Design review of the part built by this model. Coordinates are the model's own, in mm. Face numbers are marked on the shaded views. A direction names the side the tool comes from. Coordinates: 2 decimals unless noted, no trailing zeros. Loops run counter-clockwise (first coordinate to the right, second up) from the corner with the lowest first, then second, coordinate; pieces in that order, holes last. Notation, with made-up numbers: (-13, -3.75) -> (6, -3.75) arc R37 cw to (6, 32.25) -> close; hole circle Ø2 at (-17.75, 15.5). An arc over 180 degrees is marked (long way). Use one line per item in the form item = value. Start each with the question number.
1. Wall thickness on line 1 (Y direction, x = -35, z = 1.4); line 2 (X direction, y = -2.5, z = 2.5); line 3 (X direction, y = 1, z = 4.5): over which ranges is each line inside the solid? List them lowest first. Write a range as from..to.
2. Consider section A-A (z = 3.5). State the section outline as (x, y) points (3 decimals).
3. For pin 1 (5 mm diameter, centred on x = 35, y = 0, fed in from +Z); pin 2 (1.5 mm diameter, centred on y = -1.5, z = 2.5, fed in from +X); pin 3 (1.5 mm diameter, centred on x = -34, z = 3.5, fed in from +Y); pin 4 (1 mm diameter, centred on x = 17.5, z = 4.5, fed in from +Y), all flat-tipped, find the tip position at first contact; note any pin that passes through.
4. Machinability: for the marked faces 4, 5 and 6, which of the approach directions +Z, -Z, +X, -X, +Y, -Y give a long, thin tool a straight path to every point of the face, cutting with its end or side? Answer none if there is none.
5. The part is to be moulded in two halves that separate along Y. For the marked faces 1, 2 and 3, say which applies: released by +Y, released by -Y, zero draft, split by the parting line, or undercut.
6. Consider section C-C (x = -6). State the section outline as (y, z) points.
7. Consider section B-B (y = 0). State the section outline as (x, z) points (3 decimals), then the cut area to 3 significant figures.
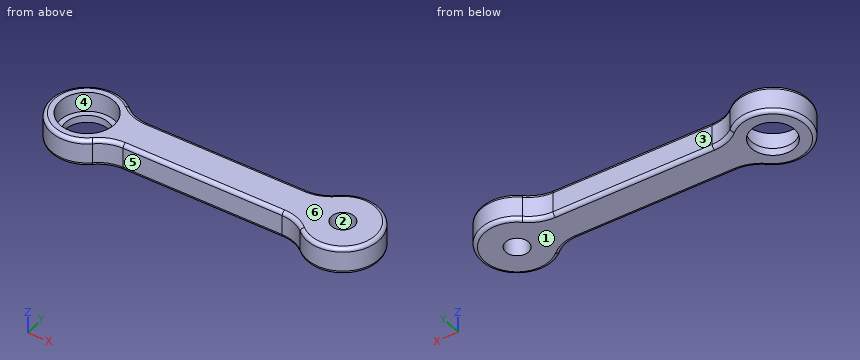
from build123d import *

# Parameters (mm, degrees)
BOSS_EXTRUDE1_DEPTH = 7.5
SKETCH2_R           = 7.5
CUT_EXTRUDE1_DEPTH  = 5.5
SKETCH3_R           = 6
CUT_EXTRUDE2_DEPTH  = 3
SKETCH4_R           = 3.175
CUT_EXTRUDE3_DEPTH  = 8.5
FILLET1_R           = 1


with BuildPart() as part:
    # Sketch1 → Boss-Extrude1 (new body)
    with BuildSketch(Plane.XY):
        with BuildLine():
            Line((-21.771243445, 5), (21.771243445, 5))
            ThreePointArc((21.771243445, 5), (25.306777351, 5.645856533), (28.385621722, 7.5))
            ThreePointArc((28.385621722, 7.5), (45, 0), (28.385621722, -7.5))
            ThreePointArc((28.385621722, -7.5), (25.306777351, -5.645856533), (21.771243445, -5))
            Line((21.771243445, -5), (-21.771243445, -5))
            ThreePointArc((-21.771243445, -5), (-25.306777351, -5.645856533), (-28.385621722, -7.5))
            ThreePointArc((-28.385621722, -7.5), (-45, 0), (-28.385621722, 7.5))
            ThreePointArc((-28.385621722, 7.5), (-25.306777351, 5.645856533), (-21.771243445, 5))
        make_face()
    extrude(amount=BOSS_EXTRUDE1_DEPTH)

    # Sketch2 → Cut-Extrude1 (cut)
    with BuildSketch(Plane.XY.offset(7.5)):
        with Locations((-35, 0)):
            Circle(SKETCH2_R)
    extrude(amount=-CUT_EXTRUDE1_DEPTH, mode=Mode.SUBTRACT)

    # Sketch3 → Cut-Extrude2 (cut, through all)
    with BuildSketch(Plane.XY.offset(2)):
        with Locations((-35, 0)):
            Circle(SKETCH3_R)
    extrude(amount=-CUT_EXTRUDE2_DEPTH, mode=Mode.SUBTRACT)

    # Sketch4 → Cut-Extrude3 (cut, through all)
    with BuildSketch(Plane(origin=(0, 0, 0), x_dir=(-1, 0, 0), z_dir=(0, 0, -1))):
        with Locations((-35, 0)):
            Circle(SKETCH4_R)
    extrude(amount=-CUT_EXTRUDE3_DEPTH, mode=Mode.SUBTRACT)

    # Fillet1
    fillet1_edges = [part.edges().sort_by_distance(p)[0] for p in [
        (25.306777351, 5.645856533, 7.5),
        (45, 0, 0),
        (25.306777351, -5.645856533, 0),
        (0, 5, 7.5),
        (-25.306777351, 5.645856533, 7.5),
        (-45, 0, 7.5),
        (-25.306777351, -5.645856533, 7.5),
        (0, -5, 7.5),
        (25.306777351, -5.645856533, 7.5),
        (45, 0, 7.5),
        (0, -5, 0),
        (-25.306777351, -5.645856533, 0),
        (-45, 0, 0),
        (-25.306777351, 5.645856533, 0),
        (0, 5, 0),
        (25.306777351, 5.645856533, 0),
    ]]
    fillet(fillet1_edges, radius=FILLET1_R)


solid = part.part
Geometry check:
q1.line_1 = -10..-6, 6..10
q1.line_2 = -44.68..-42.07, -27.93..33.04, 36.96..44.68
q1.line_3 = -44.95..-42.43, -27.57..31.99, 38.01..44.95
q2.outline = (-28.386, -7.5) arc R10 cw to (-21.771, -5) -> (21.771, -5) arc R10 cw to (28.386, -7.5) arc R10 ccw (long way) to (28.386, 7.5) arc R10 cw to (21.771, 5) -> (-21.771, 5) arc R10 cw to (-28.386, 7.5) arc R10 ccw (long way) to start; hole circle Ø15 at (-35, 0); hole circle Ø6.35 at (35, 0)
q3.pin_1 = through
q3.pin_2 = 44.97
q3.pin_3 = 10
q3.pin_4 = 5
q4.face_4 = +Z
q4.face_5 = +Z, -Z, -Y
q4.face_6 = +Z, +X, -X, +Y, -Y
q5.face_1 = zero draft
q5.face_2 = undercut
q5.face_3 = released by +Y
q6.outline = (-5, 1) arc R1 ccw to (-4, 0) -> (4, 0) arc R1 ccw to (5, 1) -> (5, 6.5) arc R1 ccw to (4, 7.5) -> (-4, 7.5) arc R1 ccw to (-5, 6.5) -> close
q7.outline = (-45, 1) arc R1 ccw to (-44, 0) -> (-41, 0) -> (-41, 2) -> (-42.5, 2) -> (-42.5, 7.5) -> (-44, 7.5) arc R1 ccw to (-45, 6.5) -> close; (-29, 0) -> (31.825, 0) -> (31.825, 7.5) -> (-27.5, 7.5) -> (-27.5, 2) -> (-29, 2) -> close; (38.175, 0) -> (44, 0) arc R1 ccw to (45, 1) -> (45, 6.5) arc R1 ccw to (44, 7.5) -> (38.175, 7.5) -> close
q7.area = 520 mm²
